Read the model definition and answer for the solid it produces. Units are mm, in the model's axes. Face numbers are marked on the shaded views. Give positions to 0.01 mm unless a question says otherwise; leave off trailing zeros. Loops run counter-clockwise (first coordinate to the right, second up) from the corner with the lowest first, then second, coordinate; pieces in that order, holes last. Notation, with made-up numbers: (89, 35) - (115, 35) arc R29 cw to (115, 59) - close; hole circle Ø6 at (3, 76.5). An arc over 180 degrees is marked (long way). Write item = value, one per line. Start each with the question number.
from build123d import *

# Parameters (mm, degrees)
SKETCH1_W                      = 673.11016
SKETCH1_H                      = 290.83
BASE_FLANGE1_DEPTH             = 3.175
EDGE_FLANGE1_DEPTH             = 351.248800168
EDGE_FLANGE2_STRIP_W           = 19.05
EDGE_FLANGE2_STRIP_H           = 3.175
EDGE_FLANGE2_STRIP_CUT_DEPTH   = 290.83
EDGE_FLANGE2_STRIP_2_W         = 19.05
EDGE_FLANGE2_STRIP_2_H         = 3.175
EDGE_FLANGE2_STRIP_CUT_2_DEPTH = 290.83
EDGE_FLANGE2_DEPTH             = 290.83
EDGE_FLANGE2_BEND_DEPTH        = 290.83


# Sheet-metal steps are written as plain solids
with BuildPart() as part:
    # Sketch1 → Base-Flange1 (new body)
    with BuildSketch(Plane(origin=(0, 0, 0), x_dir=(1, 0, 0), z_dir=(0, 1, 0))):
        with Locations((336.55508, 145.415)):
            Rectangle(SKETCH1_W, SKETCH1_H)
    extrude(amount=-BASE_FLANGE1_DEPTH)

    # Edge-Flange1 section (across the edge) → Edge-Flange1 (add)
    with BuildSketch(Plane(origin=(512.179480084, 0, -294.005), x_dir=(0, 0, 1), z_dir=(-1, 0, 0))):
        with BuildLine():
            Line((-3.175, 3.175), (-3.175, 22.225))
            Line((-3.175, 22.225), (0, 22.225))
            Line((0, 22.225), (0, 3.175))
            ThreePointArc((0, 3.175), (0.92993597, 0.92993597), (3.175, 0))
            Line((3.175, 0), (3.175, -3.175))
            ThreePointArc((3.175, -3.175), (-1.315128061, -1.315128061), (-3.175, 3.175))
        make_face()
    extrude(amount=EDGE_FLANGE1_DEPTH)

    # Edge-Flange2 strip (across the edge) → Edge-Flange2 strip cut (cut)
    with BuildSketch(Plane(origin=(673.11016, 0, 0), x_dir=(-1, 0, 0), z_dir=(0, 0, -1))):
        with Locations((-3.175, -1.5875)):
            Rectangle(EDGE_FLANGE2_STRIP_W, EDGE_FLANGE2_STRIP_H)
    extrude(amount=EDGE_FLANGE2_STRIP_CUT_DEPTH, mode=Mode.SUBTRACT)

    # Edge-Flange2 strip 2 (across the edge) → Edge-Flange2 strip cut 2 (cut)
    with BuildSketch(Plane.XY.offset(-290.83)):
        with Locations((-3.175, -1.5875)):
            Rectangle(EDGE_FLANGE2_STRIP_2_W, EDGE_FLANGE2_STRIP_2_H)
    extrude(amount=EDGE_FLANGE2_STRIP_CUT_2_DEPTH, mode=Mode.SUBTRACT)

    # Edge-Flange2 section (across the edge) → Edge-Flange2 (add)
    with BuildSketch(Plane(origin=(673.11016, 0, 0), x_dir=(-1, 0, 0), z_dir=(0, 0, -1))):
        with BuildLine():
            Line((0, 3.175), (0, 22.225))
            Line((0, 22.225), (3.175, 22.225))
            Line((3.175, 22.225), (3.175, 3.175))
            ThreePointArc((3.175, 3.175), (4.10493597, 0.92993597), (6.35, 0))
            Line((6.35, 0), (6.35, -3.175))
            ThreePointArc((6.35, -3.175), (1.859871939, -1.315128061), (0, 3.175))
        make_face()
    extrude(amount=EDGE_FLANGE2_DEPTH)

    # Edge-Flange2 section 2 (across the edge) → Edge-Flange2 bend (add)
    with BuildSketch(Plane.XY.offset(-290.83)):
        with BuildLine():
            Line((0, 3.175), (0, 22.225))
            Line((0, 22.225), (3.175, 22.225))
            Line((3.175, 22.225), (3.175, 3.175))
            ThreePointArc((3.175, 3.175), (4.10493597, 0.92993597), (6.35, 0))
            Line((6.35, 0), (6.35, -3.175))
            ThreePointArc((6.35, -3.175), (1.859871939, -1.315128061), (0, 3.175))
        make_face()
    extrude(amount=EDGE_FLANGE2_BEND_DEPTH)


solid = part.part
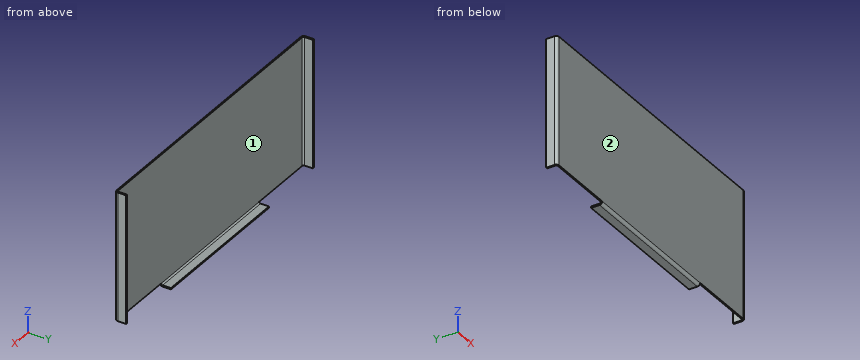
1. A cutting plane is placed at D-D on x = 612.5. Give the vertices of the cut face in (y, z) (3 decimals), and give its area (3 significant figures).
2. A cutting plane is placed at B-B on x = 331. Give the vertices of the cut face in (y, z) (3 decimals).
3. A cutting plane is placed at A-A on y = 12.5. Give the vertices of the cut face in (x, z) (3 decimals).
4. Consider line 1 along X through (y, z) = (3, -168); line 2 along Y through (x, z) = (518, -176.5) (3 decimals); line 3 along Z through (x, y) = (495, 5) (3 decimals). Determine where each line is inside the solid, lowest interval first. Write a range as [from, to].
5. For a pull along X with two mould halves and no side action, classify the marked faces 1 and 2 as released by +X, released by -X, zero draft, split by the parting line, or undercut.
6. Given P1, Ø10, axis at x = 240, y = 17, coming from the +Z side (3 decimals); P2, Ø5, axis at y = 14, z = -294.5, coming from the +X side; P3, Ø1.5, axis at x = 585.5, y = 0.5, coming from the -Z side, each flat-ended and moving along its own axis, determine where each tip first touches the part or whether it passes through.
7. A cutting plane is placed at C-C on z = -148. Give the vertices of the cut face in (x, y) (3 decimals).
Reply:
q1.outline = (-3.175, -290.83) - (0, -290.83) - (0, 0) - (-3.175, 0) - close
q1.area = 923 mm^2
q2.outline = (-3.175, -290.83) arc R6.35 ccw to (3.175, -297.18) - (22.225, -297.18) - (22.225, -294.005) - (3.175, -294.005) arc R3.175 cw to (0, -290.83) - (0, 0) - (-3.175, 0) - close
q3.outline = (0, -290.83) - (3.175, -290.83) - (3.175, 0) - (0, 0) - close; (160.931, -297.18) - (512.179, -297.18) - (512.179, -294.005) - (160.931, -294.005) - close; (669.935, -290.83) - (673.11, -290.83) - (673.11, 0) - (669.935, 0) - close
q4.line_1 = [0, 3.18], [669.93, 673.11]
q4.line_2 = [-3.175, 0]
q4.line_3 = [-297.18, -294.005]
q5.face_1 = undercut
q5.face_2 = zero draft
q6.P1 = -294.005
q6.P2 = 512.18
q6.P3 = -290.83
q7.outline = (0, 3.175) arc R6.35 ccw to (6.35, -3.175) - (666.76, -3.175) arc R6.35 ccw to (673.11, 3.175) - (673.11, 22.225) - (669.935, 22.225) - (669.935, 3.175) arc R3.175 cw to (666.76, 0) - (6.35, 0) arc R3.175 cw to (3.175, 3.175) - (3.175, 22.225) - (0, 22.225) - close
